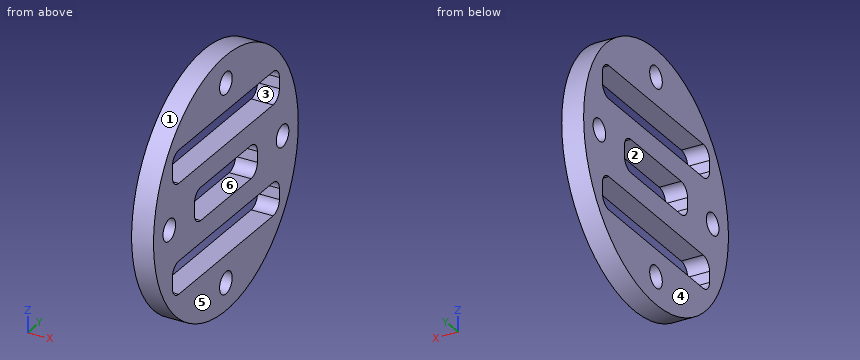
```python
from build123d import *

# Parameters (mm, degrees)
F0_R     = 11.5
F0_R_2   = 1
F0_W     = 17
F0_H     = 3
F0_W_2   = 10
F1_DEPTH = 2
F2_R     = 1


with BuildPart() as f1:
    # F0 (on Right) → F1 (new body)
    with BuildSketch(Plane.YZ):
        Circle(F0_R)
        with Locations((0, -9)):
            Circle(F0_R_2, mode=Mode.SUBTRACT)
        with Locations((0, -5)):
            Rectangle(F0_W, F0_H, mode=Mode.SUBTRACT)
        with Locations((-9, 0)):
            Circle(F0_R_2, mode=Mode.SUBTRACT)
        Rectangle(F0_W_2, F0_H, mode=Mode.SUBTRACT)
        with Locations((0, 5)):
            Rectangle(F0_W, F0_H, mode=Mode.SUBTRACT)
        with Locations((9, 0)):
            Circle(F0_R_2, mode=Mode.SUBTRACT)
        with Locations((0, 9)):
            Circle(F0_R_2, mode=Mode.SUBTRACT)
    extrude(amount=F1_DEPTH)

    # F2
    f2_edges = [f1.edges().sort_by_distance(p)[0] for p in [
        (1, -8.5, 6.5),
        (1, -8.5, 3.5),
        (1, 8.5, 6.5),
        (1, 8.5, 3.5),
        (1, 5, -1.5),
        (1, -5, -1.5),
        (1, -8.5, -6.5),
        (1, 8.5, -6.5),
        (1, -5, 1.5),
        (1, -8.5, -3.5),
        (1, 8.5, -3.5),
        (1, 5, 1.5),
    ]]
    fillet(f2_edges, radius=F2_R)


solid = f1.part
```
Could you check a few things on this model? Use its own coordinates, in mm. Face numbers are marked on the shaded views. A direction names the side the tool comes from. Give positions to 0.01 mm unless a question says otherwise; leave off trailing zeros. Loops run counter-clockwise (first coordinate to the right, second up) from the corner with the lowest first, then second, coordinate; pieces in that order, holes last. Notation, with made-up numbers: (-25.75, -7) - (32.25, -7) arc R27 ccw to (32.25, 19) - close; hole circle Ø1 at (17, -7). An arc over 180 degrees is marked (long way). Answer in a Markdown table with one row per item. Add a question column.
Q1. We'd pull the mould along Z, two halves only. Please class the marked faces 1, 2, 3 and 4: +Z half, -Z half, draft (parallel to the pull), parting line (faces both ways), or undercut.
Q2. If we section it at A-A (x = 0.9): State how many separate pieces and enclosed holes the cut face has, plus the area to 3 significant figures.
Q3. Which directions (+Z, -Z, +X, -X, +Y, -Y) give clear straight access to the entire face, cutting with the end or side of a thin tool? Please do the marked faces 5 and 6.
Q4. If we section it at B-B (z = 0): List the corners of the cut face in (x, y) for me, plus the area to 3 significant figures.
Q5. For pin 1 (0.6 mm diameter, centred on x = 1.5, y = 2, fed in from -Z); pin 2 (0.5 mm diameter, centred on x = 0.5, z = 5, fed in from +Y); pin 3 (1.2 mm diameter, centred on y = 9, z = 0, fed in from -X); pin 4 (1.1 mm diameter, centred on x = 0.5, z = -5, fed in from -Y), each with a flat end and sliding along its axis, tell me the tip position at first contact or that it passes through.
Q6. If we section it at C-C (y = 0): List the corners of the cut face in (x, z) for me, plus the area to 3 significant figures.
Q7. If we section it at D-D (y = -9.25): List the corners of the cut face in (x, z) for me, plus the area to 3 significant figures.
Q8. Please list where these lines run through material, in increasing order: L1, parallel to Z at x = 1, y = 0; L2, parallel to Z at x = 0.65, y = -6.5; L3, parallel to Z at x = 1.1, y = -4.5. Write a range as from..to.
The answers:
| question | item | result |
|---|---|---|
| 1 | face 1 | parting line |
| 1 | face 2 | undercut |
| 1 | face 3 | undercut |
| 1 | face 4 | draft |
| 2 | separate pieces | 1 |
| 2 | enclosed holes | 7 |
| 2 | area | 273 mm^2 |
| 3 | face 5 | +Z, -Z, +X, +Y, -Y |
| 3 | face 6 | +X, -X |
| 4 | outline | (0, -11.5) - (2, -11.5) - (2, -10) - (0, -10) - close; (0, -8) - (2, -8) - (2, -5) - (0, -5) - close; (0, 5) - (2, 5) - (2, 8) - (0, 8) - close; (0, 10) - (2, 10) - (2, 11.5) - (0, 11.5) - close |
| 4 | area | 18.0 mm^2 |
| 5 | pin 1 | stops at z = -11.37 |
| 5 | pin 2 | stops at y = 10.47 |
| 5 | pin 3 | passes through |
| 5 | pin 4 | stops at y = -10.6 |
| 6 | outline | (0, -11.5) - (2, -11.5) - (2, -10) - (0, -10) - close; (0, -8) - (2, -8) - (2, -6.5) - (0, -6.5) - close; (0, -3.5) - (2, -3.5) - (2, -1.5) - (0, -1.5) - close; (0, 1.5) - (2, 1.5) - (2, 3.5) - (0, 3.5) - close; (0, 6.5) - (2, 6.5) - (2, 8) - (0, 8) - close; (0, 10) - (2, 10) - (2, 11.5) - (0, 11.5) - close |
| 6 | area | 20.0 mm^2 |
| 7 | outline | (0, -6.83) - (2, -6.83) - (2, -0.97) - (0, -0.97) - close; (0, 0.97) - (2, 0.97) - (2, 6.83) - (0, 6.83) - close |
| 7 | area | 23.5 mm^2 |
| 8 | L1 | z = -11.5..-10, -8..-6.5, -3.5..-1.5, 1.5..3.5, 6.5..8, 10..11.5 |
| 8 | L2 | z = -9.49..-6.5, -3.5..3.5, 6.5..9.49 |
| 8 | L3 | z = -10.58..-6.5, -3.5..-1.37, 1.37..3.5, 6.5..10.58 |
